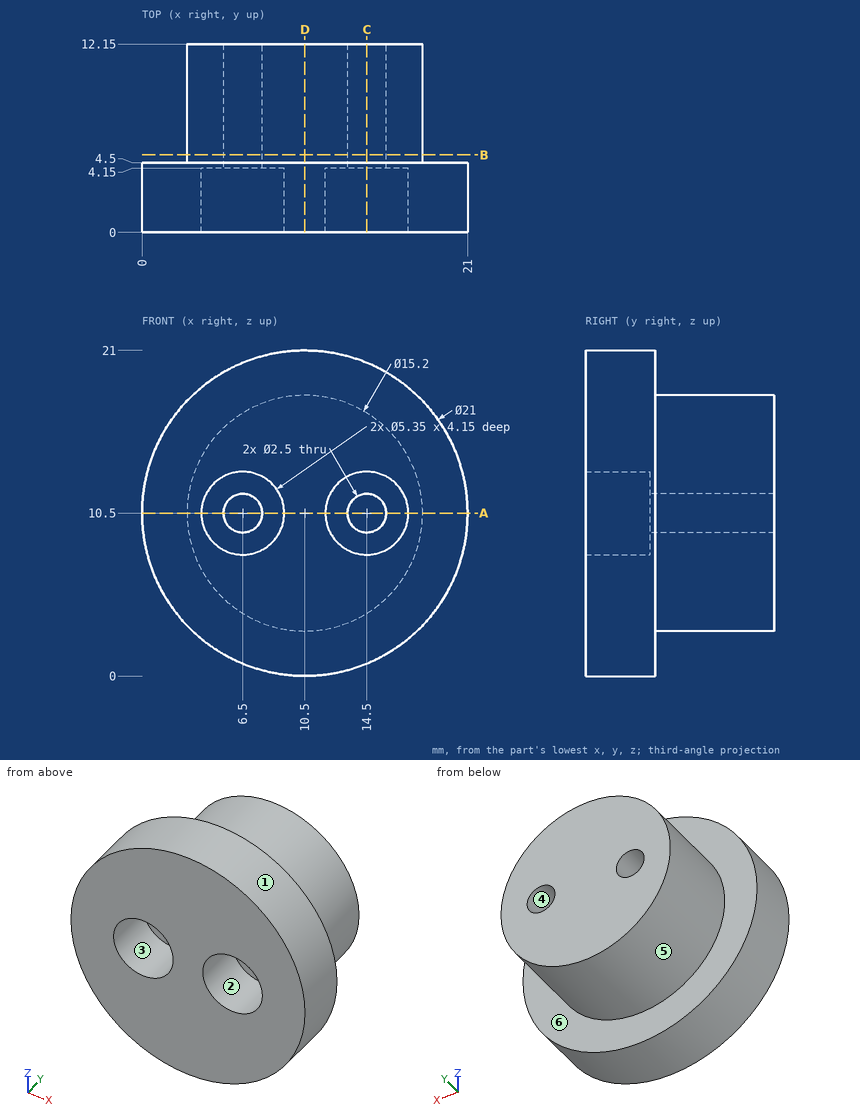
Design review of the part shown in the three views and the two pictorial views. Dimensions are in mm from the part's minimum x, y and z. A direction names the side the tool comes from. Round coordinates to 2 decimals unless told otherwise and drop trailing zeros. Write each loop counter-clockwise with the first axis right and the second up, starting at its lowest first coordinate (ties: lowest second). Pieces come first, ordered by that corner, then holes. Notation, with made-up numbers: M 3.5,35 L 28.5,35 A13 cw 28.5,44 Z; hole C 9,87.5 d11. An arc over 180 degrees is marked long. Use a Markdown table: item, result. Add a question column.
Q1. We need section B-B, the plane y = 5. State the section outline as (x, z) points.
Q2. The part is to be moulded in two halves that separate along Z. For the marked faces 3, 4, 5 and 6, say which applies: pulls with the +Z half, pulls with the -Z half, needs draft (parallel to the pull), parting line crosses it, or undercut.
Q3. To check wall thickness, follow line 1 (X direction, y = 6.75, z = 10.5); line 2 (X direction, y = 1.5, z = 12); line 3 (Y direction, x = 17.75, z = 16). State the ranges of each line that lie inside material, in increasing order.
Q4. We need section A-A, the plane z = 10.5. State the section outline as (x, y) points (3 decimals).
Q5. We need section C-C, the plane x = 14.5. State the section outline as (y, z) points (3 decimals).
Q6. We need section D-D, the plane x = 10.5. State the section outline as (y, z) points.
Q7. Machinability: for the marked faces 1 and 2, which of the approach directions +Z, -Z, +X, -X, +Y, -Y give a long, thin tool a straight path to every point of the face, cutting with its end or side? Answer none if there is none.
Q8. Insertion check: pin 1 (3 mm diameter, centred on x = 6.5, z = 10.5, fed in from -Y); pin 2 (2 mm diameter, centred on x = 7.5, y = 4.5, fed in from -Z); pin 3 (6 mm diameter, centred on x = 17, y = 7, fed in from -Z). Each pin has a flat end and moves straight along its axis. Give the tip position at first contact, or say it passes through.
Findings below:
| question | item | result |
|---|---|---|
| 1 | outline | C 10.5,10.5 d15.2; hole C 6.5,10.5 d2.5; hole C 14.5,10.5 d2.5 |
| 2 | face 3 | undercut |
| 2 | face 4 | undercut |
| 2 | face 5 | parting line crosses it |
| 2 | face 6 | needs draft |
| 3 | line 1 | x = 2.9 to 5.25, 7.75 to 13.25, 15.75 to 18.1 |
| 3 | line 2 | x = 0.11 to 4.29, 8.71 to 12.29, 16.71 to 20.89 |
| 3 | line 3 | y = 0 to 4.5 |
| 4 | outline | M 0,0 L 3.825,0 L 3.825,4.15 L 5.25,4.15 L 5.25,12.15 L 2.9,12.15 L 2.9,4.5 L 0,4.5 Z; M 7.75,4.15 L 9.175,4.15 L 9.175,0 L 11.825,0 L 11.825,4.15 L 13.25,4.15 L 13.25,12.15 L 7.75,12.15 Z; M 15.75,4.15 L 17.175,4.15 L 17.175,0 L 21,0 L 21,4.5 L 18.1,4.5 L 18.1,12.15 L 15.75,12.15 Z |
| 5 | outline | M 0,0.792 L 4.5,0.792 L 4.5,4.038 L 12.15,4.038 L 12.15,9.25 L 4.15,9.25 L 4.15,7.825 L 0,7.825 Z; M 0,13.175 L 4.15,13.175 L 4.15,11.75 L 12.15,11.75 L 12.15,16.962 L 4.5,16.962 L 4.5,20.208 L 0,20.208 Z |
| 6 | outline | M 0,0 L 4.5,0 L 4.5,2.9 L 12.15,2.9 L 12.15,18.1 L 4.5,18.1 L 4.5,21 L 0,21 Z |
| 7 | face 1 | +Y, -Y |
| 7 | face 2 | -Y |
| 8 | pin 1 | stops at y = 4.15 |
| 8 | pin 2 | stops at z = 0.19 |
| 8 | pin 3 | stops at z = 1.18 |
